Here's how the part is built. I have some questions about the finished solid (model axes, mm). A direction names the side the tool comes from. Give positions to 0.01 mm unless a question says otherwise; leave off trailing zeros. Write each loop counter-clockwise with the first axis right and the second up, starting at its lowest first coordinate (ties: lowest second). Pieces come first, ordered by that corner, then holes. Notation, with made-up numbers: (68, 8.25) - (92, 8.25) arc R28 cw to (92, 38.25) - close; hole circle Ø8 at (40, -30.5). An arc over 180 degrees is marked (long way). Write each question's results on one line, items separated by ' | '. Start each with the question number.
Item 1: Suppose I cut it at B-B on z = 2. List the corners of the cut face in (x, y) for me (3 decimals).
Item 2: Please list where these lines run through material, in increasing order: line 1 along X through (y, z) = (-1.3, -4.25); line 2 along Z through (x, y) = (-6.2, -1.95); line 3 along Z through (x, y) = (21.5, -2.7).
Item 3: We'd pull the mould along X, two halves only. Please class faces 1 (the flat face through (0, -3.175, 0)), 2 (the flat face through (23, -2, -6.579)), 3 (the flat face through (-35.089, -2, 0)): +X half, -X half, draft (parallel to the pull), parting line (faces both ways), or undercut.
Item 4: Suppose I cut it at A-A on x = -6.2. List the corners of the cut face in (y, z) for me (3 decimals).
Item 5: Suppose I cut it at C-C on y = -1.3. List the corners of the cut face in (x, z) for me.
Item 6: Which directions (+Z, -Z, +X, -X, +Y, -Y) give clear straight access to the entire face, cutting with the end or side of a thin tool? Please do faces 4 (the flat face through (-28, -2, -6.579)), 5 (the flat face through (0, 0, 0)).
```python
from build123d import *

# Parameters (mm, degrees)
F0_W     = 70.1778
F0_H     = 20.1778
F0_W_2   = 6.4122
F0_H_2   = 13.1572
F0_R     = 0.9111
F0_W_3   = 13.1572
F1_DEPTH = 3.175


with BuildPart() as f1:
    # F0 (on Front) → F1 (new body)
    with BuildSketch(Plane.XZ):
        Rectangle(F0_W, F0_H)
        with Locations((-27.495, 0)):
            Rectangle(F0_W_2, F0_H_2, mode=Mode.SUBTRACT)
        with Locations((-6.2, 0)):
            Circle(F0_R, mode=Mode.SUBTRACT)
        with Locations((22.6775, 0)):
            Rectangle(F0_W_3, F0_H_2, mode=Mode.SUBTRACT)
    extrude(amount=F1_DEPTH)


solid = f1.part
```
Checked values:
1) outline: (-35.089, -3.175) - (-30.701, -3.175) - (-30.701, 0) - (-35.089, 0) - close; (-24.289, -3.175) - (16.099, -3.175) - (16.099, 0) - (-24.289, 0) - close; (29.256, -3.175) - (35.089, -3.175) - (35.089, 0) - (29.256, 0) - close
2) line 1: x = -35.09 to -30.7, -24.29 to 16.1, 29.26 to 35.09 | line 2: z = -10.09 to -0.91, 0.91 to 10.09 | line 3: z = -10.09 to -6.58, 6.58 to 10.09
3) face 1: draft | face 2: undercut | face 3: -X half
4) outline: (-3.175, -10.089) - (0, -10.089) - (0, -0.911) - (-3.175, -0.911) - close; (-3.175, 0.911) - (0, 0.911) - (0, 10.089) - (-3.175, 10.089) - close
5) outline: (-35.09, -10.09) - (35.09, -10.09) - (35.09, 10.09) - (-35.09, 10.09) - close; hole (-30.7, -6.58) - (-24.29, -6.58) - (-24.29, 6.58) - (-30.7, 6.58) - close; hole circle Ø1.82 at (-6.2, 0); hole (16.1, -6.58) - (29.26, -6.58) - (29.26, 6.58) - (16.1, 6.58) - close
6) face 4: +Y, -Y | face 5: +Z, -Z, +X, -X, +Y
